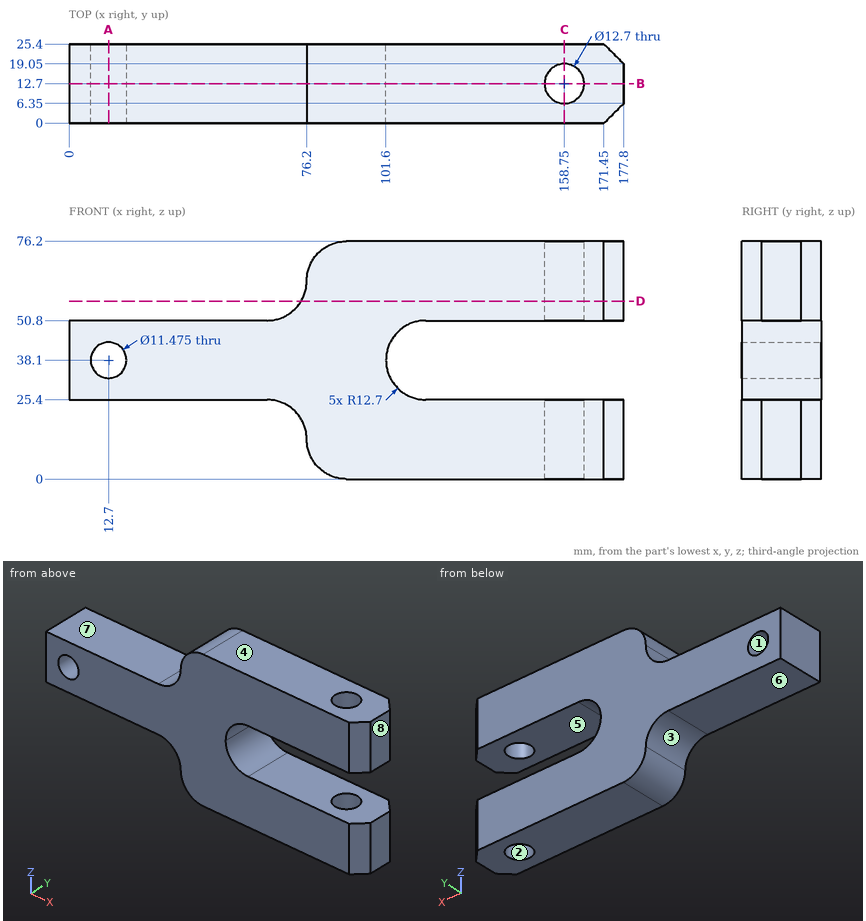
Design review of the part shown in the three views and the two pictorial views. Dimensions are in mm from the part's minimum x, y and z. A direction names the side the tool comes from. Coordinates: 2 decimals unless noted, no trailing zeros. Order: outer loops, then holes, each group sorted by start corner. A loop starts at its lowest first (then second) coordinate and runs counter-clockwise, first axis right, second up. Notation, with made-up numbers: (67.25, 38.25) -> (98.25, 38.25) arc R19 cw to (98.25, 73.25) -> close; hole circle Ø2 at (-2, 9.5). An arc over 180 degrees is marked (long way). Use one line per item in the form item = value. Start each with the question number.
(1) Add section B-B on y = 12.7. Give the number of separate pieces and of enclosed holes in the cut face, plus the area to 3 significant figures.
(2) Add section D-D on z = 57. State the section outline as (x, y) points, plus the area to 3 significant figures.
(3) For the marked faces 5, 6, 7 and 8, list the 3-axis set-ups (+Z, -Z, +X, -X, +Y, -Y) from which the entire face can be reached by the end or side of a thin tool; tool diameter is ignored.
(4) Add section A-A on x = 12.7. State the section outline as (y, z) points.
(5) Insertion check: pin 1 (1.5 mm diameter, centred on x = 18.5, y = 15.5, fed in from +Z); pin 2 (12.5 mm diameter, centred on x = 46, y = 15.5, fed in from -Z); pin 3 (3 mm diameter, centred on y = 18, z = 34.5, fed in from +X). Each pin has a flat end and moves straight along its axis. Give the tip position at first contact, or say it passes through.
(6) The part is to be moulded in two halves that separate along X. For the marked faces 1, 2, 3 and 4, say which applies: +X half, -X half, draft (parallel to the pull), parting line (faces both ways), or undercut.
(7) Add section C-C on x = 158.75. State the section outline as (y, z) points.
(8) For probe 1 along Z at (x, y) = (125.5, 11.5); probe 2 along Y at (x, z) = (158.75, 14.75); probe 3 along Z at (x, y) = (52, 20.5), list the stretches that pass through material, from the lowest coordinate up.
Answer block:
q1.separate_pieces = 3
q1.enclosed_holes = 1
q1.area = 7,060 mm²
q2.outline = (74.41, 0) -> (171.45, 0) -> (177.8, 6.35) -> (177.8, 19.05) -> (171.45, 25.4) -> (74.41, 25.4) -> close; hole circle Ø12.7 at (158.75, 12.7)
q2.area = 2,460 mm²
q3.face_5 = +X, +Y, -Y
q3.face_6 = -Z, -X, +Y, -Y
q3.face_7 = +Z, -X, +Y, -Y
q3.face_8 = +Z, -Z, +X, +Y, -Y
q4.outline = (0, 25.4) -> (25.4, 25.4) -> (25.4, 32.36) -> (0, 32.36) -> close; (0, 43.84) -> (25.4, 43.84) -> (25.4, 50.8) -> (0, 50.8) -> close
q5.pin_1 = 50.8
q5.pin_2 = 25.4
q5.pin_3 = 102.67
q6.face_1 = undercut
q6.face_2 = undercut
q6.face_3 = -X half
q6.face_4 = draft
q7.outline = (0, 0) -> (6.35, 0) -> (6.35, 25.4) -> (0, 25.4) -> close; (0, 50.8) -> (6.35, 50.8) -> (6.35, 76.2) -> (0, 76.2) -> close; (19.05, 0) -> (25.4, 0) -> (25.4, 25.4) -> (19.05, 25.4) -> close; (19.05, 50.8) -> (25.4, 50.8) -> (25.4, 76.2) -> (19.05, 76.2) -> close
q8.probe_1 = 0 to 25.4, 50.8 to 76.2
q8.probe_2 = 0 to 6.35, 19.05 to 25.4
q8.probe_3 = 25.4 to 50.8
